from build123d import *

# Parameters (mm, degrees)
BOSS_EXTRUDE1_DEPTH = 0.94


with BuildPart() as part:
    # Sketch2 → Boss-Extrude1 (new body)
    with BuildSketch(Plane.XY):
        with BuildLine():
            Line((7.944739921, 2.128786646), (8.862369456, 2.374664739))
            Line((8.862369456, 2.374664739), (9.779998991, 2.620542832))
            ThreePointArc((9.779998991, 2.620542832), (-10.077153498, 0.983159385), (9.089055299, -4.46146823))
            ThreePointArc((9.089055299, -4.46146823), (8.698265252, -3.448205084), (8.862369456, -2.374664739))
            Line((8.862369456, -2.374664739), (7.944739921, -2.128786646))
            ThreePointArc((7.944739921, -2.128786646), (-8.225, 0), (7.944739921, 2.128786646))
        make_face()
    extrude(amount=BOSS_EXTRUDE1_DEPTH)


solid = part.part
CAD build for the part. Positions are in the model's coordinates, mm. A direction names the side the tool comes from. Give positions to 0.01 mm unless a question says otherwise; leave off trailing zeros. Write each loop counter-clockwise with the first axis right and the second up, starting at its lowest first coordinate (ties: lowest second). Pieces come first, ordered by that corner, then holes. Notation, with made-up numbers: M 64.5,-28 L 120.5,-28 A13 cw 120.5,-18 Z; hole C 58.5,41 d10. An arc over 180 degrees is marked long. Put each result on its own line as item: value. Start each with the question number.
(1) Band-saw the part on C-C, the plane y = 5.25. Write the cut outline in (x, z), and give its area (3 significant figures).
(2) Flat gauge pins, fed straight in: pin 1 Ø6 at (x, y) = (-6, 7) entering from -Z; pin 2 Ø1.5 at (x, y) = (-3.5, 6.5) entering from +Z. Where does each tip first touch, or does it go through?
(3) Band-saw the part on D-D, the plane y = 0. Write the cut outline in (x, z) (3 decimals), and give its area (3 significant figures).
(4) Probe L1, parallel to Y at x = 0, z = 0.7 (3 decimals); L2, parallel to X at y = 0, z = 0.45 (3 decimals); L3, parallel to Y at x = 5.5, z = 0.15. List the from-to ranges inside material, lowest first.
(5) Which spindle directions (+Z, -Z, +X, -X, +Y, -Y) get a long thin tool onto all of the face, cutting with end or side? Do faces 4 (the face through (8.85, 2.37, 0.46)), 5 (the face through (-8.3, -1.5, 0)). Say none if no direction does.
(6) Band-saw the part on A-A, the plane x = 0. Write the cut outline in (y, z) (3 decimals), and give its area (3 significant figures).
(7) Band-saw the part on B-B, the plane z = 0.3. Write the cut outline in (x, y) (3 decimals).
(8) Mould opens along Y. For faces 1 (the face through (8.41, -2.253, 0.463)), 2 (the face through (-10.03, 1.37, 0.46)), 3 (the face through (-8.3, -1.5, 0.94)) say: +Y half, -Y half, draft (parallel to the pull), parting line (faces both ways), or undercut.
Response values:
1. outline: M -8.66,0 L -6.33,0 L -6.33,0.94 L -8.66,0.94 Z; M 6.33,0 L 8.66,0 L 8.66,0.94 L 6.33,0.94 Z
1. area: 4.37 mm2
2. pin 1: stops at z = 0
2. pin 2: passes through
3. outline: M -10.125,0 L -8.225,0 L -8.225,0.94 L -10.125,0.94 Z
3. area: 1.79 mm2
4. L1: y = -10.125 to -8.225, 8.225 to 10.125
4. L2: x = -10.125 to -8.225
4. L3: y = -8.5 to -6.12, 6.12 to 8.5
5. face 4: +Z, -Z, +X
5. face 5: -Z, +X, -X, +Y, -Y
6. outline: M -10.125,0 L -8.225,0 L -8.225,0.94 L -10.125,0.94 Z; M 8.225,0 L 10.125,0 L 10.125,0.94 L 8.225,0.94 Z
6. area: 3.57 mm2
7. outline: M 7.945,-2.129 A8.225 cw long 7.945,2.129 L 9.78,2.621 A10.125 ccw long 9.089,-4.461 A2.113 cw 8.862,-2.375 Z
8. face 1: undercut
8. face 2: parting line
8. face 3: draft
